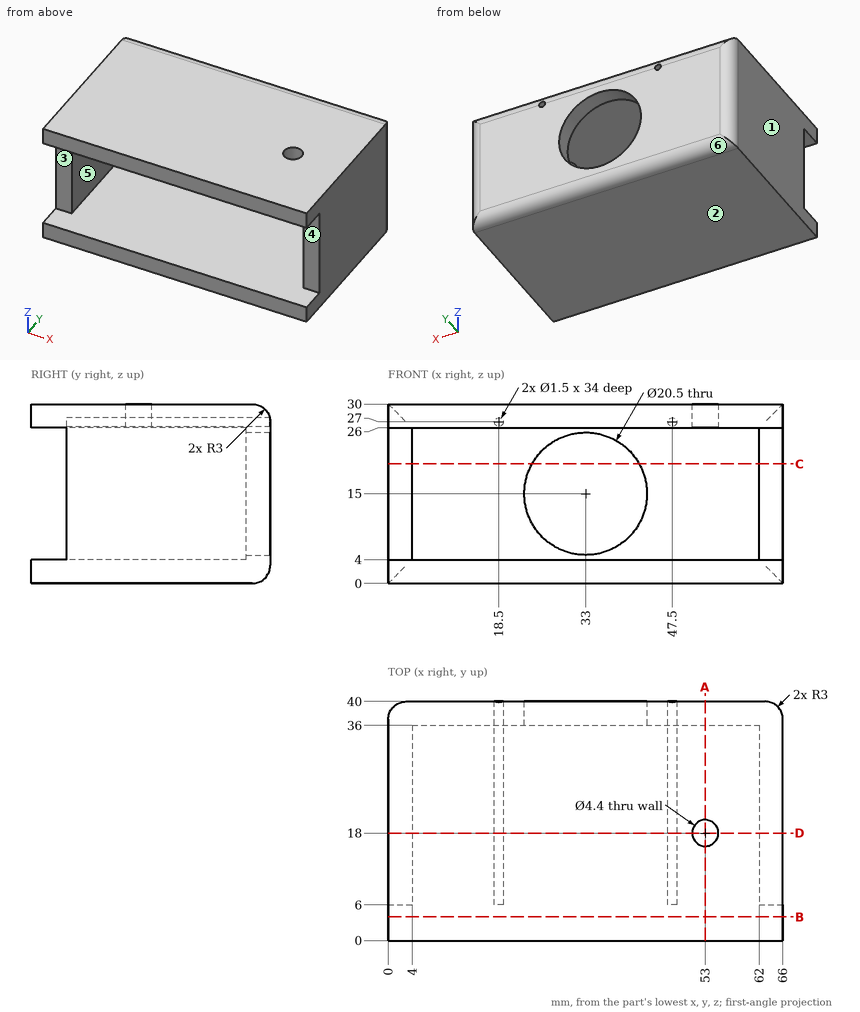
Verification items for this drawing (mm, ordinates from the low corner). A direction names the side the tool comes from. Give positions to 0.01 mm unless a question says otherwise; leave off trailing zeros. Write each loop counter-clockwise with the first axis right and the second up, starting at its lowest first coordinate (ties: lowest second). Pieces come first, ordered by that corner, then holes.
1) Release check for a two-part mould opening along Z. For the marked faces 1, 2 and 3 record: released by +Z, released by -Z, zero draft, split by the parting line, or undercut.
Values follow:
face 1: zero draft
face 2: released by -Z
face 3: undercut
2) Cross-section at D-D (y = 18). Record the boundary of the cut face in (x, z).
Values follow:
outline: (0, 0) - (66, 0) - (66, 30) - (55.2, 30) - (55.2, 26) - (62, 26) - (62, 4) - (4, 4) - (4, 26) - (50.8, 26) - (50.8, 30) - (0, 30) - close; hole circle Ø1.5 at (18.5, 27); hole circle Ø1.5 at (47.5, 27)
3) Cross-section at C-C (z = 20). Record the boundary of the cut face in (x, y).
Values follow:
outline: (0, 6) - (4, 6) - (4, 36) - (24.05, 36) - (24.05, 40) - (3, 40) arc R3 ccw to (0, 37) - close; (41.95, 36) - (62, 36) - (62, 6) - (66, 6) - (66, 37) arc R3 ccw to (63, 40) - (41.95, 40) - close
4) Thickness scan on line 1 (Z direction, x = 47.5, y = 19); line 2 (Z direction, x = 33.5, y = 10.5); line 3 (X direction, y = 35, z = 14.5). Record the ranges inside material, lowest first.
Values follow:
line 1: z = 0 to 4, 26 to 26.25, 27.75 to 30
line 2: z = 0 to 4, 26 to 30
line 3: x = 0 to 4, 62 to 66
5) Go/stop test with flat-tipped pins: pin 1 Ø4 at (x, y) = (53, 18) entering from +Z; pin 2 Ø1.4 at (x, z) = (47.5, 27) entering from -Y; pin 3 Ø12.5 at (x, z) = (33, 15) entering from +Y; pin 4 Ø4.5 at (x, z) = (64.5, 15.5) entering from -Y. Record where each tip stops, or that it passes through.
Values follow:
pin 1: stops at z = 4
pin 2: stops at y = 0
pin 3: passes through
pin 4: stops at y = 6
6) Cross-section at B-B (y = 4). Record the boundary of the cut face in (x, z).
Values follow:
outline: (0, 0) - (66, 0) - (66, 4) - (0, 4) - close; (0, 26) - (66, 26) - (66, 30) - (0, 30) - close
7) Set-up check for the marked faces 4, 5 and 6: record each of +Z, -Z, +X, -X, +Y, -Y from which the full face is reachable in a straight line by a thin tool's end or side.
Values follow:
face 4: +X, -X, -Y
face 5: -Y
face 6: -Z, +X, -X, +Y
8) Cross-section at A-A (x = 53). Record the boundary of the cut face in (y, z).
Values follow:
outline: (0, 0) - (37, 0) arc R3 ccw to (40, 3) - (40, 27) arc R3 ccw to (37, 30) - (20.2, 30) - (20.2, 26) - (36, 26) - (36, 4) - (0, 4) - close; (0, 26) - (15.8, 26) - (15.8, 30) - (0, 30) - close
